from build123d import *

# Parameters (mm, degrees)
SKETCH_1_W          = 15
SKETCH_1_H          = 15
SKETCH_1_W_2        = 12
SKETCH_1_H_2        = 12
EXTRUDE_2_DEPTH     = 750
SKETCH_3_R          = 2.15
CUT_EXTRUDE_1_DEPTH = 751.187476568
SKETCH_4_R          = 2.15
CUT_EXTRUDE_2_DEPTH = 751.187476568


with BuildPart() as part:
    # ｽｹｯﾁ1 → 押し出し-薄板2 (new body)
    with BuildSketch(Plane.XY):
        Rectangle(SKETCH_1_W, SKETCH_1_H)
        Rectangle(SKETCH_1_W_2, SKETCH_1_H_2, mode=Mode.SUBTRACT)
    extrude(amount=EXTRUDE_2_DEPTH)

    # ｽｹｯﾁ3 → ｶｯﾄ - 押し出し1 (cut, through all)
    with BuildSketch(Plane(origin=(0, 7.5, 0), x_dir=(1, 0, 0), z_dir=(0, 1, 0))):
        with Locations(Location((0, -745, 0), (0, 0, 270))):
            Circle(SKETCH_3_R)
        with Locations(Location((0, -5, 0), (0, 0, 270))):
            Circle(SKETCH_3_R)
        with Locations(Location((0, -490, 0), (0, 0, 270))):
            Circle(SKETCH_3_R)
        with Locations(Location((0, -460, 0), (0, 0, 270))):
            Circle(SKETCH_3_R)
        with Locations(Location((0, -570, 0), (0, 0, 270))):
            Circle(SKETCH_3_R)
        with Locations(Location((0, -290, 0), (0, 0, 270))):
            Circle(SKETCH_3_R)
        with Locations(Location((0, -260, 0), (0, 0, 270))):
            Circle(SKETCH_3_R)
        with Locations(Location((0, -70, 0), (0, 0, 270))):
            Circle(SKETCH_3_R)
        with Locations(Location((0, -440, 0), (0, 0, 270))):
            Circle(SKETCH_3_R)
    extrude(amount=-CUT_EXTRUDE_1_DEPTH, mode=Mode.SUBTRACT)

    # ｽｹｯﾁ4 → ｶｯﾄ - 押し出し2 (cut, through all)
    with BuildSketch(Plane(origin=(7.5, 0, 0), x_dir=(0, 0, -1), z_dir=(1, 0, 0))):
        with Locations(Location((-360, 0, 0), (0, 0, 90))):
            Circle(SKETCH_4_R)
        with Locations(Location((-390, 0, 0), (0, 0, 90))):
            Circle(SKETCH_4_R)
        with Locations(Location((-375, 0, 0), (0, 0, 90))):
            Circle(SKETCH_4_R)
        with Locations(Location((-732.5, 0, 0), (0, 0, 90))):
            Circle(SKETCH_4_R)
        with Locations(Location((-17.5, 0, 0), (0, 0, 90))):
            Circle(SKETCH_4_R)
        with Locations(Location((-420, 0, 0), (0, 0, 90))):
            Circle(SKETCH_4_R)
        with Locations(Location((-330, 0, 0), (0, 0, 90))):
            Circle(SKETCH_4_R)
        with Locations(Location((-663, 2, 0), (0, 0, 90))):
            Circle(SKETCH_4_R)
        with Locations(Location((-93.5, 0, 0), (0, 0, 90))):
            Circle(SKETCH_4_R)
    extrude(amount=-CUT_EXTRUDE_2_DEPTH, mode=Mode.SUBTRACT)


solid = part.part
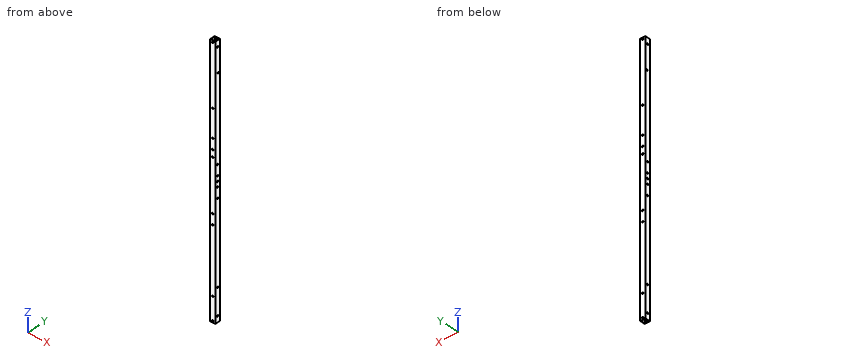
The listing builds one solid part. Answer for the finished solid, in the listing's coordinates (mm). Coordinates: 2 decimals unless noted, no trailing zeros. Write each loop counter-clockwise with the first axis right and the second up, starting at its lowest first coordinate (ties: lowest second). Pieces come first, ordered by that corner, then holes. Notation, with made-up numbers: M 44,-26 L 65,-26 A10 ccw 65,-21 Z; hole C -39.75,49.25 d6. An arc over 180 degrees is marked long. Put each result on its own line as item: value. Start each with the question number.
1. Consider line 1 (X direction, y = -6.65, z = 440); line 2 (X direction, y = -5, z = 433). Determine where each line is inside the solid, lowest interval first. Write a range as from..to.
2. A flat-ended cylindrical pin translates along its axis: P1, Ø2.5, axis at y = 0, z = 360, coming from the -X side. Find the tip coordinate at first contact, or state that the pin passes through.
3. A cutting plane is placed at A-A on z = 508.5. Write down the section's boundary in (x, y), then the cut area to 3 significant figures.
Resolved:
1. line 1: x = -7.5..-2.15, 2.15..7.5
1. line 2: x = -7.5..-6, 6..7.5
2. P1: passes through
3. outline: M -7.5,-7.5 L 7.5,-7.5 L 7.5,7.5 L -7.5,7.5 Z; hole M -6,-6 L 6,-6 L 6,6 L -6,6 Z
3. area: 81.0 mm2
